Check sheet for the modelled part. Datum: model origin and axes. Units: mm. Round coordinates to 2 decimals unless told otherwise and drop trailing zeros. Loops run counter-clockwise (first coordinate to the right, second up) from the corner with the lowest first, then second, coordinate; pieces in that order, holes last. Notation, with made-up numbers: (-10.5, 53) - (12.5, 53) arc R6 ccw to (12.5, 57) - close; hole circle Ø6 at (1, 82). An arc over 180 degrees is marked (long way). Put each result on its own line as item: value. Start each with the question number.
Item 1: Section check A-A, the plane x = 2.95. Record the cut outline in (y, z), and give its area (3 significant figures).
Item 2: Gauge pin test, flat ends, axial feed: pin 1 Ø8 at (y, z) = (-29.5, 35.5) entering from -X; pin 2 Ø1.5 at (x, y) = (1.5, 321) entering from +Z; pin 3 Ø1.5 at (x, y) = (3, 32) entering from -Z. Record the tip position at first contact, or that the pin passes through.
Item 3: Section check D-D, the plane z = 74. Record the cut outline in (x, y).
Item 4: Material ranges on line 1 along Z through (x, y) = (1.75, 268); line 2 along Y through (x, z) = (1.5, 70); line 3 along Y through (x, z) = (0.75, 66), recorded low to high.
Item 5: Section check B-B, the plane z = 48. Record the cut outline in (x, y), and give its area (3 significant figures).
Item 6: Section check C-C, the plane y = 101.5. Record the cut outline in (x, z), and give its area (3 significant figures).
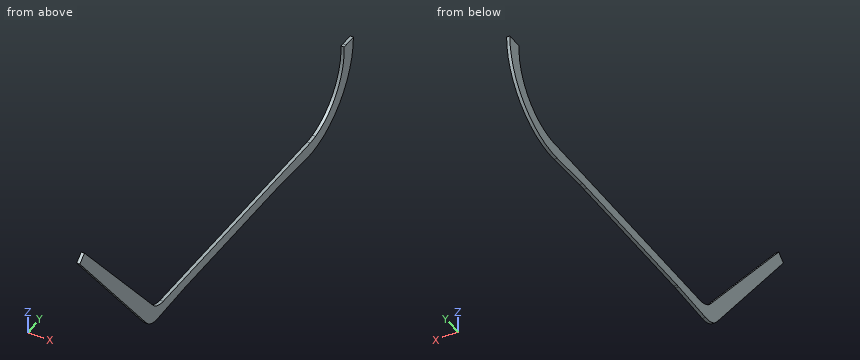
from build123d import *

# Parameters (mm, degrees)
F1_DEPTH = 4


# Not quite as in the source:
# - a feature names something its author has since deleted; it is built from what else it names


with BuildPart() as f1:
    # F0 (on Right) → F1 (new body)
    with BuildSketch(Plane.YZ):
        with BuildLine():
            Line((-151.036893852, 186.5150307497), (-7.0347090015, 8.6871421429))
            ThreePointArc((-7.0347090015, 8.6871421429), (4.1862889829, 0.1122435093), (18.0871758973, -2.3787453176))
            Line((18.0871758973, -2.3787453176), (76.0584955576, -0.0786202013))
            ThreePointArc((76.0584955576, -0.0786202013), (78.0403935877, -0.0196569823), (80.023071087, 0))
            Line((80.023071087, 0), (275.0031210998, 0))
            ThreePointArc((275.0031210998, 0), (279.998441154, -0.0623927883), (284.9906444886, -0.2495322244))
            Line((284.9906444886, -0.2495322244), (340, -3))
            ThreePointArc((340, -3), (412.2291799256, 23.705892636), (442.8144690376, 94.379786148))
            Line((442.8144690376, 94.379786148), (426.8144690376, 94.448943804))
            Line((426.8144690376, 94.448943804), (422.8144690376, 94.448943804))
            ThreePointArc((422.8144690376, 94.448943804), (406.6400435708, 42.8631388402), (360.6700266042, 14.4120430259))
            ThreePointArc((360.6700266042, 14.4120430259), (355.0395932087, 13.5090940512), (349.3599875605, 13))
            Line((349.3599875605, 13), (29.918677403, 13))
            ThreePointArc((29.918677403, 13), (17.4430940609, 15.7170415777), (7.2272892953, 23.3760119817))
            Line((7.2272892953, 23.3760119817), (-140.933996353, 194.6961958333))
            Line((-140.933996353, 194.6961958333), (-151.036893852, 186.5150307497))
        make_face()
    extrude(amount=F1_DEPTH)


solid = f1.part
Check result:
1. outline: (-151.04, 186.52) - (-7.03, 8.69) arc R30 ccw to (18.09, -2.38) - (76.06, -0.08) arc R100 cw to (80.02, 0) - (275, 0) arc R200 cw to (284.99, -0.25) - (340, -3) arc R97.93 ccw to (442.81, 94.38) - (426.81, 94.45) - (422.81, 94.45) arc R77.48 cw to (360.67, 14.41) arc R81.93 cw to (349.36, 13) - (29.92, 13) arc R30 cw to (7.23, 23.38) - (-140.93, 194.7) - close
1. area: 11,100 mm²
2. pin 1: x = 0
2. pin 2: z = 13
2. pin 3: z = -1.86
3. outline: (0, -59.92) - (4, -59.92) - (4, -36.55) - (0, -36.55) - close; (0, 421.17) - (4, 421.17) - (4, 440.58) - (0, 440.58) - close
4. line 1: 0 to 13
4. line 2: -56.68 to -33.09, 420.19 to 439.62
4. line 3: -53.45 to -29.63, 418.99 to 438.48
5. outline: (0, -38.87) - (4, -38.87) - (4, -14.07) - (0, -14.07) - close; (0, 410.3) - (4, 410.3) - (4, 430.91) - (0, 430.91) - close
5. area: 182 mm²
6. outline: (0, 0) - (4, 0) - (4, 13) - (0, 13) - close
6. area: 52.0 mm²
